Read the model definition and answer for the solid it produces. Units are mm, in the model's axes. Face numbers are marked on the shaded views. A direction names the side the tool comes from. Coordinates: 2 decimals unless noted, no trailing zeros. Loops run counter-clockwise (first coordinate to the right, second up) from the corner with the lowest first, then second, coordinate; pieces in that order, holes last. Notation, with made-up numbers: M 58.25,78 L 71.25,78 A32 cw 71.25,113 Z; hole C 44.5,54.5 d4. An arc over 180 degrees is marked long. Put each result on its own line as item: value.
from build123d import *

# Parameters (mm, degrees)
SKETCH_W        = 326
SKETCH_H        = 146
PAD_DEPTH       = 24
SKETCH001_W     = 320
SKETCH001_H     = 138
POCKET_DEPTH    = 10
POCKET001_DEPTH = 350
SKETCH003_W     = 312
SKETCH003_H     = 130
POCKET002_DEPTH = 10
SKETCH004_W     = 312
SKETCH004_H     = 2
PAD001_DEPTH    = 8
POCKET003_DEPTH = 1
POCKET004_DEPTH = 1
SKETCH007_W     = 326
SKETCH007_H     = 24
PAD002_DEPTH    = 10
PAD003_DEPTH    = 20
PAD004_DEPTH    = 20
POCKET005_DEPTH = 160
POCKET006_DEPTH = 380
POCKET007_DEPTH = 360
FILLET_R        = 1
FILLET001_R     = 1
FILLET002_R     = 1
FILLET003_R     = 1
FILLET004_R     = 1
FILLET005_R     = 1
FILLET006_R     = 1
FILLET007_R     = 1
FILLET008_R     = 2
FILLET009_R     = 2
FILLET010_R     = 2
FILLET011_R     = 2
FILLET012_R     = 2
FILLET013_R     = 2
FILLET014_R     = 2
FILLET015_R     = 2


with BuildPart() as part:
    # Sketch → Pad (new body)
    with BuildSketch(Plane.XY):
        with Locations((163, -73)):
            Rectangle(SKETCH_W, SKETCH_H)
    extrude(amount=PAD_DEPTH)

    # Sketch001 (on Face5 of Pad) → Pocket (cut)
    with BuildSketch(Plane(origin=(0, 0, 0), x_dir=(1, 0, 0), z_dir=(0, 0, -1))):
        with Locations((163, 72)):
            Rectangle(SKETCH001_W, SKETCH001_H)
    extrude(amount=-POCKET_DEPTH, mode=Mode.SUBTRACT)

    # Sketch002 (on Face2 of Pocket) → Pocket001 (cut)
    with BuildSketch(Plane(origin=(0, 0, 0), x_dir=(0, -1, 0), z_dir=(-1, 0, 0))):
        Polygon((0, 0), (146, 0), (146, 8), align=None)
    extrude(amount=-POCKET001_DEPTH, mode=Mode.SUBTRACT)

    # Sketch003 (on Face11 of Pocket001) → Pocket002 (cut)
    with BuildSketch(Plane(origin=(0, 0, 10), x_dir=(1, 0, 0), z_dir=(0, 0, -1))):
        with Locations((163, 72)):
            Rectangle(SKETCH003_W, SKETCH003_H)
    extrude(amount=-POCKET002_DEPTH, mode=Mode.SUBTRACT)

    # Sketch004 (on Face16 of Pocket002) → Pad001 (join)
    with BuildSketch(Plane(origin=(0, 0, 20), x_dir=(1, 0, 0), z_dir=(0, 0, -1))):
        with Locations((163, 37)):
            Rectangle(SKETCH004_W, SKETCH004_H)
    extrude(amount=PAD001_DEPTH)

    # Sketch005 (on Face5 of Pad001) → Pocket003 (cut)
    with BuildSketch(Plane.XY.offset(24)):
        with BuildLine():
            add(Edge.make_bspline(
                [(197.39, -37.25), (194.95, -10.73), (163.08, 3.81), (137.21, -26.19)],
                knots=[0, 0, 0, 0, 1, 1, 1, 1], degree=3))
            add(Edge.make_bspline(
                [(137.21, -26.19), (110.49, -21.03), (106.38, -47.47)],
                knots=[0, 0, 0, 1, 1, 1], degree=2))
            add(Edge.make_bspline(
                [(106.38, -47.47), (77.83, -55.23), (78.31, -100.02), (112.19, -99.1)],
                knots=[0, 0, 0, 0, 1, 1, 1, 1], degree=3))
            Line((112.19, -99.1), (198.8, -99.1))
            add(Edge.make_bspline(
                [(197.39, -37.25), (247.04, -44.58), (238.66, -96.16), (198.8, -99.1)],
                knots=[0, 0, 0, 0, 1, 1, 1, 1], degree=3))
        make_face()
    extrude(amount=-POCKET003_DEPTH, mode=Mode.SUBTRACT)

    # Sketch006 (on Face5 of Pocket003) → Pocket004 (cut)
    with BuildSketch(Plane.XY.offset(24)):
        with BuildLine():
            add(Edge.make_bspline(
                [(134.29, -105.39), (118.6, -116.37), (120.88, -135.91), (137.06, -131.62), (140.99, -119.42), (139.96, -102.27), (134.29, -105.39)],
                knots=[0, 0, 0, 0, 0.25, 0.5, 0.75, 1, 1, 1, 1], degree=3))
        make_face()
        with BuildLine():
            add(Edge.make_bspline(
                [(157.29, -105.39), (141.6, -116.37), (143.88, -135.91), (160.06, -131.62), (163.99, -119.42), (162.96, -102.27), (157.29, -105.39)],
                knots=[0, 0, 0, 0, 0.25, 0.5, 0.75, 1, 1, 1, 1], degree=3))
        make_face()
        with BuildLine():
            add(Edge.make_bspline(
                [(180.29, -105.39), (164.6, -116.37), (166.88, -135.91), (183.06, -131.62), (186.99, -119.42), (185.96, -102.27), (180.29, -105.39)],
                knots=[0, 0, 0, 0, 0.25, 0.5, 0.75, 1, 1, 1, 1], degree=3))
        make_face()
    extrude(amount=-POCKET004_DEPTH, mode=Mode.SUBTRACT)

    # Sketch007 (on Face1 of Pocket004) → Pad002 (join)
    with BuildSketch(Plane(origin=(0, 0, 0), x_dir=(-1, 0, 0), z_dir=(0, 1, 0))):
        with Locations((-163, 12)):
            Rectangle(SKETCH007_W, SKETCH007_H)
    extrude(amount=PAD002_DEPTH)

    # Sketch009 (on Face1 of Pad002) → Pad003 (join)
    with BuildSketch(Plane(origin=(0, 0, 0), x_dir=(0, -1, 0), z_dir=(-1, 0, 0))):
        Polygon((-10, 24), (-10, 0), (0, 0), (146, 8), (146, 24), align=None)
    extrude(amount=PAD003_DEPTH)

    # Sketch010 (on Face4 of Pad003) → Pad004 (join)
    with BuildSketch(Plane.YZ.offset(326)):
        Polygon((10, 24), (10, 0), (0, 0), (-146, 8), (-146, 24), align=None)
    extrude(amount=PAD004_DEPTH)

    # Sketch011 (on Face19 of Pad004) → Pocket005 (cut)
    with BuildSketch(Plane(origin=(0, 10, 0), x_dir=(-1, 0, 0), z_dir=(0, 1, 0))):
        Polygon((10, 0), (0, 24), (62.814814, 43.289979), (90.06, 0), align=None)
    extrude(amount=-POCKET005_DEPTH, mode=Mode.SUBTRACT)

    # Sketch012 (on Face30 of Pocket005) → Pocket006 (cut)
    with BuildSketch(Plane(origin=(0, 10, 0), x_dir=(-1, 0, 0), z_dir=(0, 1, 0))):
        Polygon((-383.56, 0), (-336, 0), (-326, 24), (-386.967866, 53.431433), align=None)
    extrude(amount=-POCKET006_DEPTH, mode=Mode.SUBTRACT)

    # Sketch013 → Pocket007 (cut, symmetric)
    with BuildSketch(Plane.YZ):
        Polygon((0, 0), (3.1, 56.61), (76.09231, 25.718735), (62.818003, -34.69), align=None)
    extrude(amount=POCKET007_DEPTH, both=True, mode=Mode.SUBTRACT)

    # Fillet
    fillet_edges = [part.edges().sort_by_distance(p)[0] for p in [
        (0, 0.657128, 24),
    ]]
    fillet(fillet_edges, radius=FILLET_R)

    # Fillet001
    fillet001_edges = [part.edges().sort_by_distance(p)[0] for p in [
        (163.333333, 1.314255, 24),
    ]]
    fillet(fillet001_edges, radius=FILLET001_R)

    # Fillet002
    fillet002_edges = [part.edges().sort_by_distance(p)[0] for p in [
        (326, -73, 24),
    ]]
    fillet(fillet002_edges, radius=FILLET002_R)

    # Fillet003
    fillet003_edges = [part.edges().sort_by_distance(p)[0] for p in [
        (329.461538, -146, 15.692308),
    ]]
    fillet(fillet003_edges, radius=FILLET003_R)

    # Fillet004
    fillet004_edges = [part.edges().sort_by_distance(p)[0] for p in [
        (163, -3, 10),
    ]]
    fillet(fillet004_edges, radius=FILLET004_R)

    # Fillet005
    fillet005_edges = [part.edges().sort_by_distance(p)[0] for p in [
        (323, -72.5, 10),
    ]]
    fillet(fillet005_edges, radius=FILLET005_R)

    # Fillet006
    fillet006_edges = [part.edges().sort_by_distance(p)[0] for p in [
        (162.5, -141, 10),
    ]]
    fillet(fillet006_edges, radius=FILLET006_R)

    # Fillet007
    fillet007_edges = [part.edges().sort_by_distance(p)[0] for p in [
        (3, -72, 10),
    ]]
    fillet(fillet007_edges, radius=FILLET007_R)

    # Fillet008
    fillet008_edges = [part.edges().sort_by_distance(p)[0] for p in [
        (163, -7, 20),
    ]]
    fillet(fillet008_edges, radius=FILLET008_R)

    # Fillet009
    fillet009_edges = [part.edges().sort_by_distance(p)[0] for p in [
        (319, -7, 14),
    ]]
    fillet(fillet009_edges, radius=FILLET009_R)

    # Fillet010
    fillet010_edges = [part.edges().sort_by_distance(p)[0] for p in [
        (162, -36, 20),
    ]]
    fillet(fillet010_edges, radius=FILLET010_R)

    # Fillet011
    fillet011_edges = [part.edges().sort_by_distance(p)[0] for p in [
        (7, -21.5, 20),
    ]]
    fillet(fillet011_edges, radius=FILLET011_R)

    # Fillet012
    fillet012_edges = [part.edges().sort_by_distance(p)[0] for p in [
        (319, -38, 16),
    ]]
    fillet(fillet012_edges, radius=FILLET012_R)

    # Fillet013
    fillet013_edges = [part.edges().sort_by_distance(p)[0] for p in [
        (319, -88.5, 20),
    ]]
    fillet(fillet013_edges, radius=FILLET013_R)

    # Fillet014
    fillet014_edges = [part.edges().sort_by_distance(p)[0] for p in [
        (162, -137, 20),
    ]]
    fillet(fillet014_edges, radius=FILLET014_R)

    # Fillet015
    fillet015_edges = [part.edges().sort_by_distance(p)[0] for p in [
        (7, -87.5, 20),
    ]]
    fillet(fillet015_edges, radius=FILLET015_R)


solid = part.part
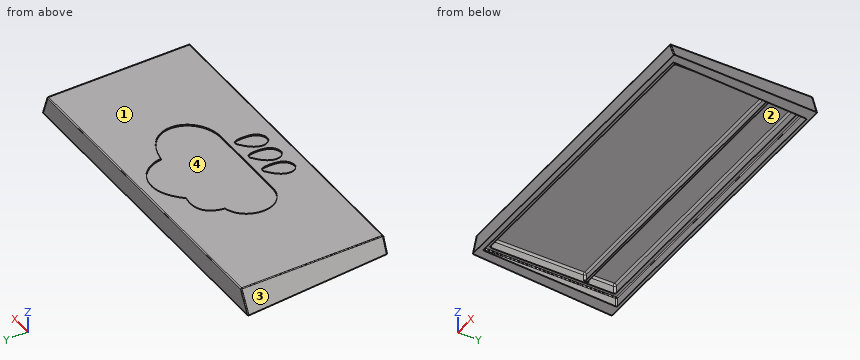
1) Determine the mould class of the marked faces 3 and 4 for opening direction Y: released by +Y, released by -Y, zero draft, split by the parting line, or undercut.
Answer list:
face 3: zero draft
face 4: undercut
2) Given pin 1 Ø20 at (x, y) = (173.5, -15.5) entering from -Z; pin 2 Ø2 at (x, z) = (53.5, 8) entering from +Y; pin 3 Ø3 at (x, y) = (108, -37.5) entering from -Z, each flat-ended and moving along its own axis, determine where each tip first touches the part or whether it passes through.
Answer list:
pin 1: stops at z = 10
pin 2: stops at y = 0.49
pin 3: stops at z = 12
3) Straight lines are drawn through the part: line 1 (X direction, y = -62.5, z = 10.75); line 2 (Y direction, x = 25, z = 16.5); line 3 (Z direction, x = 269.5, y = -93.5). For each, find the intervals that lie inside material, in ascending order. Write a range as [from, to].
Answer list:
line 1: x = [-5.52, 7], [319, 331.52]
line 2: y = [-146, -137], [-38, -36], [-7, 0.9]
line 3: z = [20, 24]
4) Which of the six approach directions +Z, -Z, +X, -X, +Y, -Y give full straight-line access (tool end or side, diameter ignored) to the marked faces 1 and 2?
Answer list:
face 1: +Z, +X, -X, +Y, -Y
face 2: -Z
5) Find section A-A, the plane x = 42. Write down the section's boundary in (y, z).
Answer list:
outline: M -146,8 L -141,7.73 L -141,9 A1 cw -140,10 L -137,10 L -137,18 A2 cw -135,20 L -40,20 A2 cw -38,18 L -38,12 L -36,12 L -36,18 A2 cw -34,20 L -9,20 A2 cw -7,18 L -7,10 L -4,10 A1 cw -3,9 L -3,0.16 L 0,0 L 1.26,22.95 A1 ccw 0.26,24 L -145,24 A1 ccw -146,23 Z
